from build123d import *

# Parameters (mm, degrees)
EXTRUDE_1_DEPTH     = 15
SKETCH_3_R          = 4.25
CUT_EXTRUDE_1_DEPTH = 44.058100283
SKETCH_5_R          = 1
CUT_EXTRUDE_2_DEPTH = 46


with BuildPart() as part:
    # 草图1 → 凸台-拉伸1 (new, symmetric)
    with BuildSketch(Plane.XY):
        Polygon((0, -30), (0, 0), (30, 0), (30, -3), (3, -3), (3, -30), align=None)
    extrude(amount=EXTRUDE_1_DEPTH, both=True)

    # 草图3 → 切除-拉伸1 (cut, through all)
    with BuildSketch(Plane(origin=(3, 0, 0), x_dir=(0, 0, -1), z_dir=(1, 0, 0))):
        with Locations((0, -15)):
            Circle(SKETCH_3_R)
    extrude(amount=-CUT_EXTRUDE_1_DEPTH, mode=Mode.SUBTRACT)

    # 草图5 → 切除-拉伸2 (cut, through all)
    with BuildSketch(Plane(origin=(0, 0, 0), x_dir=(1, 0, 0), z_dir=(0, 1, 0))):
        with Locations(Location((15, 0, 0), (0, 0, 270))):
            Circle(SKETCH_5_R)
    extrude(amount=-CUT_EXTRUDE_2_DEPTH, mode=Mode.SUBTRACT)


solid = part.part
The model under review builds one solid part; all positions refer to its coordinate system, in mm. A direction names the side the tool comes from. Give positions to 0.01 mm unless a question says otherwise; leave off trailing zeros. Order: outer loops, then holes, each group sorted by start corner. A loop starts at its lowest first (then second) coordinate and runs counter-clockwise, first axis right, second up. Notation, with made-up numbers: (72, 11.5) -> (106, 11.5) arc R20 cw to (106, 16.5) -> close; hole circle Ø5 at (-18, -9.5). An arc over 180 degrees is marked (long way). Write item = value, one per line. Start each with the question number.
(1) Take a section at D-D (x = 26.5). Write out the cut boundary in (y, z), plus the area to 3 significant figures.
(2) Take a section at B-B (x = 15). Write out the cut boundary in (y, z).
(3) For L1, parallel to X at y = -2.3, z = 0; L2, parallel to Y at x = 1.95, z = 0; L3, parallel to Y at x = 3.75, z = 1.75, list the stretches that pass through material, from the lowest coordinate up. Write a range as from..to.
(4) Take a section at C-C (z = 11.5). Write out the cut boundary in (x, y), plus the area to 3 significant figures.
(5) Tool access review of faces 4 (the flat face through (30, -1, 0)), 5 (the flat face through (3, -19, 4)): name each direction out of +Z, -Z, +X, -X, +Y, -Y from which nothing blocks a thin tool from reaching the whole face with its end or side.
(6) Draft analysis for pull direction X (two halves, no side actions). For faces 1 (the flat face through (0, -19, 4)), 2 (the flat face through (2, -30, 0)), 3 (the cylindrical face through (14, -1, 0)), state which applies: +X half, -X half, draft (parallel to the pull), parting line (faces both ways), or undercut.
(7) For pin 1 Ø5 at (y, z) = (-19.5, -3.5) entering from +X; pin 2 Ø1.2 at (x, z) = (15, 0) entering from -Y; pin 3 Ø6 at (y, z) = (-17.5, 8) entering from -X, all flat-tipped, find the tip position at first contact; note any pin that passes through.
(8) Take a section at A-A (y = -15). Write out the cut boundary in (x, z).
Returned:
q1.outline = (-3, -15) -> (0, -15) -> (0, 15) -> (-3, 15) -> close
q1.area = 90.0 mm²
q2.outline = (-3, -15) -> (0, -15) -> (0, -1) -> (-3, -1) -> close; (-3, 1) -> (0, 1) -> (0, 15) -> (-3, 15) -> close
q3.L1 = 0..14, 16..30
q3.L2 = -30..-19.25, -10.75..0
q3.L3 = -3..0
q4.outline = (0, -30) -> (3, -30) -> (3, -3) -> (30, -3) -> (30, 0) -> (0, 0) -> close
q4.area = 171 mm²
q5.face_4 = +Z, -Z, +X, +Y, -Y
q5.face_5 = +Z, -Z, +X, -Y
q6.face_1 = -X half
q6.face_2 = draft
q6.face_3 = undercut
q7.pin_1 = 3
q7.pin_2 = through
q7.pin_3 = 0
q8.outline = (0, -15) -> (3, -15) -> (3, -4.25) -> (0, -4.25) -> close; (0, 4.25) -> (3, 4.25) -> (3, 15) -> (0, 15) -> close
